```python
from build123d import *

# Parameters (mm, degrees)
BOSS_EXTRUDE1_DEPTH = 8.8
BOSS_EXTRUDE3_DEPTH = 8.8


with BuildPart() as part:
    # Sketch1 → Boss-Extrude1 (new body)
    with BuildSketch(Plane(origin=(0, 0, 0), x_dir=(0, 0, -1), z_dir=(1, 0, 0))):
        Polygon((0, 0), (15, 5.459553514), (15, 0), align=None)
    extrude(amount=BOSS_EXTRUDE1_DEPTH)

    # Sketch2 → Boss-Extrude3 (add)
    with BuildSketch(Plane.ZY):
        with BuildLine():
            Line((-15, 5.459553514), (-14.289665454, 5.201012883))
            ThreePointArc((-14.289665454, 5.201012883), (-14.585776352, 5.492539256), (-15, 5.459553514))
        make_face()
        with BuildLine():
            Line((-14.248245903, 5.185937399), (-13.537911358, 4.927396768))
            ThreePointArc((-13.537911358, 4.927396768), (-13.834022255, 5.218923141), (-14.248245903, 5.185937399))
        make_face()
        with BuildLine():
            Line((-13.496491807, 4.912321285), (-12.786157261, 4.653780654))
            ThreePointArc((-12.786157261, 4.653780654), (-13.082268159, 4.945307027), (-13.496491807, 4.912321285))
        make_face()
        with BuildLine():
            Line((-12.74473771, 4.63870517), (-12.034403164, 4.380164539))
            ThreePointArc((-12.034403164, 4.380164539), (-12.330514062, 4.671690912), (-12.74473771, 4.63870517))
        make_face()
        with BuildLine():
            Line((-11.992983613, 4.365089055), (-11.282649068, 4.106548424))
            ThreePointArc((-11.282649068, 4.106548424), (-11.578759965, 4.398074797), (-11.992983613, 4.365089055))
        make_face()
        with BuildLine():
            Line((-11.241229517, 4.091472941), (-10.530894971, 3.83293231))
            ThreePointArc((-10.530894971, 3.83293231), (-10.827005869, 4.124458683), (-11.241229517, 4.091472941))
        make_face()
        with BuildLine():
            Line((-10.48947542, 3.817856826), (-9.779140875, 3.559316195))
            ThreePointArc((-9.779140875, 3.559316195), (-10.075251772, 3.850842568), (-10.48947542, 3.817856826))
        make_face()
        with BuildLine():
            Line((-9.737721324, 3.544240711), (-9.027386778, 3.28570008))
            ThreePointArc((-9.027386778, 3.28570008), (-9.323497675, 3.577226453), (-9.737721324, 3.544240711))
        make_face()
        with BuildLine():
            Line((-8.985967227, 3.270624597), (-8.275632681, 3.012083966))
            ThreePointArc((-8.275632681, 3.012083966), (-8.571743579, 3.303610339), (-8.985967227, 3.270624597))
        make_face()
        with BuildLine():
            Line((-8.23421313, 2.997008482), (-7.523878585, 2.738467851))
            ThreePointArc((-7.523878585, 2.738467851), (-7.819989482, 3.029994224), (-8.23421313, 2.997008482))
        make_face()
        with BuildLine():
            Line((-7.482459034, 2.723392367), (-6.772124488, 2.464851736))
            ThreePointArc((-6.772124488, 2.464851736), (-7.068235386, 2.756378109), (-7.482459034, 2.723392367))
        make_face()
        with BuildLine():
            Line((-6.730704937, 2.449776253), (-6.020370391, 2.191235622))
            ThreePointArc((-6.020370391, 2.191235622), (-6.316481289, 2.482761995), (-6.730704937, 2.449776253))
        make_face()
        with BuildLine():
            Line((-5.97895084, 2.176160138), (-5.268616295, 1.917619507))
            ThreePointArc((-5.268616295, 1.917619507), (-5.564727192, 2.20914588), (-5.97895084, 2.176160138))
        make_face()
        with BuildLine():
            Line((-5.227196744, 1.902544023), (-4.516862198, 1.644003392))
            ThreePointArc((-4.516862198, 1.644003392), (-4.812973096, 1.935529765), (-5.227196744, 1.902544023))
        make_face()
        with BuildLine():
            Line((-4.475442647, 1.628927909), (-3.765108101, 1.370387278))
            ThreePointArc((-3.765108101, 1.370387278), (-4.061218999, 1.661913651), (-4.475442647, 1.628927909))
        make_face()
        with BuildLine():
            Line((-3.723688551, 1.355311794), (-3.013354005, 1.096771163))
            ThreePointArc((-3.013354005, 1.096771163), (-3.309464902, 1.388297536), (-3.723688551, 1.355311794))
        make_face()
        with BuildLine():
            Line((-2.971934454, 1.081695679), (-2.261599908, 0.823155048))
            ThreePointArc((-2.261599908, 0.823155048), (-2.557710806, 1.114681421), (-2.971934454, 1.081695679))
        make_face()
        with BuildLine():
            Line((-2.220180357, 0.808079565), (-1.509845812, 0.549538934))
            ThreePointArc((-1.509845812, 0.549538934), (-1.805956709, 0.841065307), (-2.220180357, 0.808079565))
        make_face()
        with BuildLine():
            Line((-1.468426261, 0.53446345), (-0.758091715, 0.275922819))
            ThreePointArc((-0.758091715, 0.275922819), (-1.054202613, 0.567449192), (-1.468426261, 0.53446345))
        make_face()
        with BuildLine():
            Line((-0.716672164, 0.260847335), (-0.006337618, 0.002306704))
            ThreePointArc((-0.006337618, 0.002306704), (-0.302448516, 0.293833077), (-0.716672164, 0.260847335))
        make_face()
    extrude(amount=-BOSS_EXTRUDE3_DEPTH)


solid = part.part
```
The listing builds one solid part. Answer for the finished solid, in the listing's coordinates (mm). Coordinates: 2 decimals unless noted, no trailing zeros. Loops run counter-clockwise (first coordinate to the right, second up) from the corner with the lowest first, then second, coordinate; pieces in that order, holes last. Notation, with made-up numbers: (14, 58) -> (23, 58) arc R9 cw to (23, 62) -> close; hole circle Ø8 at (1, -38.75). An arc over 180 degrees is marked (long way). Return JSON: item names as keys, results as strings. Group by question number.
(1) Given pin 1 Ø4 at (x, z) = (8, -12) entering from -Y; pin 2 Ø1.5 at (y, z) = (4.5, -4.5) entering from -X; pin 3 Ø5 at (x, z) = (5, -10.5) entering from +Y, each flat-ended and moving along its own axis, determine where each tip first touches the part or whether it passes through.
(2) A cutting plane is placed at B-B on z = -13.75. Write down the section's boundary in (x, y).
(3) A cutting plane is placed at A-A on z = -11.75. Write down the section's boundary in (x, y).
(4) Find the intervals of material crossed by probe 1 along Y at (x, z) = (5.25, -5); probe 2 along Y at (x, z) = (6.5, -10.5); probe 3 along Z at (x, y) = (7, 4.55), in increasing order. Write a range as from..to.
The answers:
{
 "1": {"pin 1": "stops at y = 0", "pin 2": "passes through", "pin 3": "stops at y = 4.91"},
 "2": {"outline": "(0, 0) -> (8.8, 0) -> (8.8, 5.18) -> (0, 5.18) -> close"},
 "3": {"outline": "(0, 0) -> (8.8, 0) -> (8.8, 4.43) -> (0, 4.43) -> close"},
 "4": {"probe 1": "y = 0..1.97", "probe 2": "y = 0..3.82", "probe 3": "z = -15..-12.14"}
}
